Can you work these out from the model? Positions are in its coordinate system, mm. Face numbers are marked on the shaded views. A direction names the side the tool comes from. Give positions to 0.01 mm unless a question says otherwise; leave off trailing zeros. Order: outer loops, then holes, each group sorted by start corner. A loop starts at its lowest first (then second) coordinate and runs counter-clockwise, first axis right, second up. Notation, with made-up numbers: (22.25, -30) -> (45.25, -30) arc R20 cw to (45.25, -17) -> close; hole circle Ø1 at (-3, 69). An arc over 180 degrees is marked (long way). Answer as a JSON object with one key per item and string values.
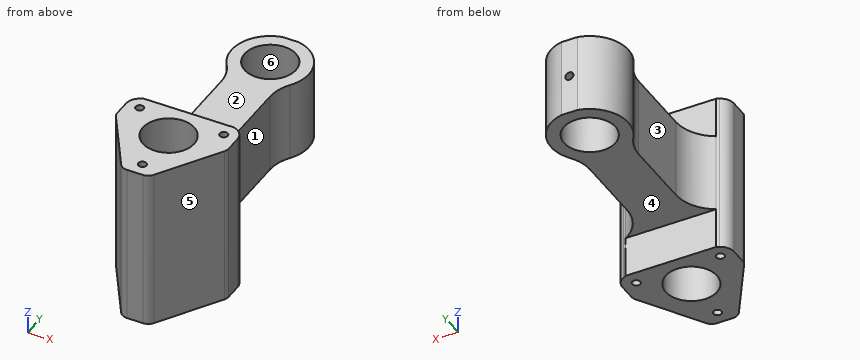
```python
from build123d import *

# Parameters (mm, degrees)
BOSS_EXTRUDE1_DEPTH = 25
SKETCH1_3_R         = 7.9375
BOSS_EXTRUDE2_DEPTH = 12.3
SKETCH3_R           = 1.25
CUT_EXTRUDE1_DEPTH  = 12.672784854
SKETCH4_R           = 1.25
CUT_EXTRUDE2_DEPTH  = 10
SKETCH5_R           = 7.9375
CUT_EXTRUDE3_DEPTH  = 51


with BuildPart() as part:
    # Sketch1 → Boss-Extrude1 (new body, symmetric)
    with BuildSketch(Plane.XY):
        with BuildLine():
            Line((14.011631608, -46.463203436), (-14.011631608, -46.463203436))
            ThreePointArc((-14.011631608, -46.463203436), (-14.401354266, -46.671858143), (-14.798102621, -46.866822962))
            ThreePointArc((-14.798102621, -46.866822962), (-16.578229761, -48.435081034), (-17.240381057, -50.713203436))
            Line((-17.240381057, -50.713203436), (-17.240381057, -55.713203436))
            ThreePointArc((-17.240381057, -55.713203436), (-17.123784168, -56.541446455), (-16.783056724, -57.305309102))
            Line((-16.783056724, -57.305309102), (-5.042675667, -76.055309102))
            ThreePointArc((-5.042675667, -76.055309102), (-3.953217637, -77.087733584), (-2.5, -77.463203436))
            Line((-2.5, -77.463203436), (2.5, -77.463203436))
            ThreePointArc((2.5, -77.463203436), (3.953217637, -77.087733584), (5.042675667, -76.055309102))
            Line((5.042675667, -76.055309102), (16.783056724, -57.305309102))
            ThreePointArc((16.783056724, -57.305309102), (17.123784168, -56.541446455), (17.240381057, -55.713203436))
            Line((17.240381057, -55.713203436), (17.240381057, -50.713203436))
            ThreePointArc((17.240381057, -50.713203436), (16.578229761, -48.435081034), (14.798102621, -46.866822962))
            ThreePointArc((14.798102621, -46.866822962), (14.401354266, -46.671858143), (14.011631608, -46.463203436))
        make_face()
    extrude(amount=BOSS_EXTRUDE1_DEPTH, both=True)

    # Sketch1_3 → Boss-Extrude2 (add, symmetric)
    with BuildSketch(Plane.XY):
        with BuildLine():
            Line((-17.240381057, -50.713203436), (-17.240381057, -55.713203436))
            ThreePointArc((-17.240381057, -55.713203436), (-17.123784168, -56.541446455), (-16.783056724, -57.305309102))
            Line((-16.783056724, -57.305309102), (-5.042675667, -76.055309102))
            ThreePointArc((-5.042675667, -76.055309102), (-3.953217637, -77.087733584), (-2.5, -77.463203436))
            Line((-2.5, -77.463203436), (2.5, -77.463203436))
            ThreePointArc((2.5, -77.463203436), (3.953217637, -77.087733584), (5.042675667, -76.055309102))
            Line((5.042675667, -76.055309102), (16.783056724, -57.305309102))
            ThreePointArc((16.783056724, -57.305309102), (17.123784168, -56.541446455), (17.240381057, -55.713203436))
            Line((17.240381057, -55.713203436), (17.240381057, -50.713203436))
            ThreePointArc((17.240381057, -50.713203436), (16.578229761, -48.435081034), (14.798102621, -46.866822962))
            ThreePointArc((14.798102621, -46.866822962), (9.478663873, -42.180498841), (7.5, -35.372933076))
            Line((7.5, -35.372933076), (7.5, -14.105545231))
            ThreePointArc((7.5, -14.105545231), (8.085343648, -10.294364118), (9.787417555, -6.83449807))
            ThreePointArc((9.787417555, -6.83449807), (11.107431649, 4.373656183), (2.5, 11.672784854))
            Line((2.5, 11.672784854), (-2.5, 11.672784854))
            ThreePointArc((-2.5, 11.672784854), (-11.107431649, 4.373656183), (-9.787417555, -6.83449807))
            ThreePointArc((-9.787417555, -6.83449807), (-8.085343648, -10.294364118), (-7.5, -14.105545231))
            Line((-7.5, -14.105545231), (-7.5, -35.372933076))
            ThreePointArc((-7.5, -35.372933076), (-9.478663873, -42.180498841), (-14.798102621, -46.866822962))
            ThreePointArc((-14.798102621, -46.866822962), (-16.578229761, -48.435081034), (-17.240381057, -50.713203436))
        make_face()
        Circle(SKETCH1_3_R, mode=Mode.SUBTRACT)
    extrude(amount=BOSS_EXTRUDE2_DEPTH, both=True)

    # Sketch3 → Cut-Extrude1 (cut, through all)
    with BuildSketch(Plane(origin=(0, 0, 0), x_dir=(1, 0, 0), z_dir=(0, 1, 0))):
        Circle(SKETCH3_R)
    extrude(amount=CUT_EXTRUDE1_DEPTH, mode=Mode.SUBTRACT)

    # Sketch4 → Cut-Extrude2 (cut)
    with BuildSketch(Plane.XY.offset(25)):
        with Locations((-12.990381057, -50.713203436)):
            Circle(SKETCH4_R)
        with Locations((12.990381057, -50.713203436)):
            Circle(SKETCH4_R)
        with Locations((0, -73.213203436)):
            Circle(SKETCH4_R)
    cut_extrude2 = extrude(amount=-CUT_EXTRUDE2_DEPTH, mode=Mode.SUBTRACT)

    # Mirror1: Cut-Extrude2 across plane
    add(cut_extrude2.mirror(Plane.XY), mode=Mode.SUBTRACT)

    # Sketch5 → Cut-Extrude3 (cut, through all)
    with BuildSketch(Plane.XY.offset(25)):
        with Locations((0, -58.213203436)):
            Circle(SKETCH5_R)
    extrude(amount=-CUT_EXTRUDE3_DEPTH, mode=Mode.SUBTRACT)


solid = part.part
```
1. If we section it at D-D on z = -8: Count the separate pieces of the cut face and the enclosed holes in it, then the cut area to 3 significant figures.
Worked answers:
{"separate pieces": "1", "enclosed holes": "2", "area": "1,410 mm²"}
2. For the marked faces 1, 2 and 3, which set-ups out of +Z, -Z, +X, -X, +Y, -Y let a thin tool reach every point of the face, with its end or its side?
Worked answers:
{"face 1": "+Z, -Z, +X", "face 2": "+Z, +X, -X, +Y", "face 3": "+Z, -Z, -X"}
3. If we section it at B-B on x = 0: Please give me the cut outline in (y, z).
Worked answers:
{"outline": "(-77.46, -25) -> (-74.46, -25) -> (-74.46, -15) -> (-71.96, -15) -> (-71.96, -25) -> (-66.15, -25) -> (-66.15, 25) -> (-71.96, 25) -> (-71.96, 15) -> (-74.46, 15) -> (-74.46, 25) -> (-77.46, 25) -> close; (-50.28, -25) -> (-46.46, -25) -> (-46.46, -12.3) -> (-7.94, -12.3) -> (-7.94, 12.3) -> (-46.46, 12.3) -> (-46.46, 25) -> (-50.28, 25) -> close; (7.94, -12.3) -> (11.67, -12.3) -> (11.67, -1.25) -> (7.94, -1.25) -> close; (7.94, 1.25) -> (11.67, 1.25) -> (11.67, 12.3) -> (7.94, 12.3) -> close"}
4. If we section it at A-A on y = 0: Please give me the cut outline in (x, z).
Worked answers:
{"outline": "(-11.94, -12.3) -> (-7.94, -12.3) -> (-7.94, 12.3) -> (-11.94, 12.3) -> close; (7.94, -12.3) -> (11.94, -12.3) -> (11.94, 12.3) -> (7.94, 12.3) -> close"}
5. Please list where these lines run through material, in increasing order: L1, parallel to Y at x = 0, z = -18.25; L2, parallel to Y at x = 3.5, z = 3; L3, parallel to Z at x = 4.5, y = -36.
Worked answers:
{"L1": "-77.46 to -74.46, -71.96 to -66.15, -50.28 to -46.46", "L2": "-77.29 to -65.34, -51.09 to -7.12, 7.12 to 11.41", "L3": "-12.3 to 12.3"}
6. Will these pins go through, and if not, where does the flat tip stop? pin 1 Ø4 at (x, z) = (4, 21) entering from +Y; pin 2 Ø2 at (x, y) = (12.99, -50.71) entering from +Z; pin 3 Ø2 at (x, y) = (12.99, -50.71) entering from -Z.
Worked answers:
{"pin 1": "y = -46.46", "pin 2": "z = 15", "pin 3": "z = -15"}
7. If we mould it in two halves opening along Y, with no side actions, what happens to the marked faces 4, 5 and 6? For each: +Y half, -Y half, draft (parallel to the pull), parting line (faces both ways), or undercut.
Worked answers:
{"face 4": "draft", "face 5": "-Y half", "face 6": "undercut"}
